Build history of the part. All positions in model axes, mm. A direction names the side the tool comes from. Coordinates: 2 decimals unless noted, no trailing zeros. Write each loop counter-clockwise with the first axis right and the second up, starting at its lowest first coordinate (ties: lowest second). Pieces come first, ordered by that corner, then holes.
```python
from build123d import *
from build123d.topology import SkipClean

# Parameters (mm, degrees)
SKETCH_1_R          = 12.5
EXTRUDE_1_DEPTH     = 4
SKETCH_2_R          = 1
EXTRUDE_2_DEPTH     = 7.5
SKETCH_5_R          = 6
CUT_EXTRUDE_1_DEPTH = 10
CUT_EXTRUDE_START   = -7.5
SKETCH_7_R          = 1
CUT_EXTRUDE_2_DEPTH = 7.5
SKETCH_8_R          = 12.5
SKETCH_8_R_2        = 6
CUT_EXTRUDE_3_DEPTH = 10
SKETCH_9_R          = 1
EXTRUDE_3_DEPTH     = 10
CUT_EXTRUDE_START_2 = -14
SKETCH_10_R         = 1
CUT_EXTRUDE_4_DEPTH = 14
SKETCH_11_R         = 8
CUT_EXTRUDE_5_DEPTH = 10
EXTRUDE_START       = -10
SKETCH_12_R         = 8
EXTRUDE_4_DEPTH     = 10
SKETCH_14_R         = 8
CUT_EXTRUDE_6_DEPTH = 10
SKETCH_15_W         = 0.086708075
SKETCH_15_H         = 4
SKETCH_16_R         = 0.7
CUT_EXTRUDE_7_DEPTH = 10
SKETCH_18_R         = 12.5
EXTRUDE_5_DEPTH     = 2.07
CUT_EXTRUDE_START_3 = -2.07
SKETCH_20_R         = 8
CUT_EXTRUDE_8_DEPTH = 2.07


with BuildPart() as part:
    # 草图1 → 凸台-拉伸1 (new body)
    with BuildSketch(Plane(origin=(0, 0, 0), x_dir=(1, 0, 0), z_dir=(0, 1, 0))):
        with Locations(Location((0, 0, 0), (0, 0, 270))):
            Circle(SKETCH_1_R)
    extrude(amount=EXTRUDE_1_DEPTH)

    # 草图2 → 凸台-拉伸2 (add)
    with BuildSketch(Plane(origin=(0, 4, 0), x_dir=(1, 0, 0), z_dir=(0, 1, 0))):
        with Locations(Location((10, 0, 0), (0, 0, 270))):
            Circle(SKETCH_2_R)
        with Locations(Location((3.399186938, -10.461621679, 0), (0, 0, 270))):
            Circle(SKETCH_2_R)
        with Locations(Location((-8.590169944, -7.416694292, 0), (0, 0, 270))):
            Circle(SKETCH_2_R)
        with Locations(Location((-9.399186938, 4.926796007, 0), (0, 0, 270))):
            Circle(SKETCH_2_R)
        with Locations(Location((2.090169944, 9.510565163, 0), (0, 0, 270))):
            Circle(SKETCH_2_R)
    extrude(amount=EXTRUDE_2_DEPTH)

    # 草图5 → 切除-拉伸1 (cut)
    with BuildSketch(Plane(origin=(0, 4, 0), x_dir=(1, 0, 0), z_dir=(0, 1, 0))):
        with Locations(Location((0, 0, 0), (0, 0, 270))):
            Circle(SKETCH_5_R)
    extrude(amount=-CUT_EXTRUDE_1_DEPTH, mode=Mode.SUBTRACT)

    # 草图7 → 切除-拉伸2 (cut)
    with BuildSketch(Plane(origin=(0, 11.5, 0), x_dir=(1, 0, 0), z_dir=(0, 1, 0)).offset(CUT_EXTRUDE_START)):
        with Locations((-9.399186938, 4.926796007)):
            Circle(SKETCH_7_R)
    extrude(amount=CUT_EXTRUDE_2_DEPTH, mode=Mode.SUBTRACT)

    # 草图8 → 切除-拉伸3 (cut)
    with BuildSketch(Plane(origin=(0, 4, 0), x_dir=(1, 0, 0), z_dir=(0, 1, 0))):
        with Locations(Location((0, 0, 0), (0, 0, 270))):
            Circle(SKETCH_8_R)
        with Locations(Location((0, 0, 0), (0, 0, 270))):
            Circle(SKETCH_8_R_2, mode=Mode.SUBTRACT)
    extrude(amount=CUT_EXTRUDE_3_DEPTH, mode=Mode.SUBTRACT)

    # 草图9 → 凸台-拉伸3 (add)
    with BuildSketch(Plane(origin=(0, 4, 0), x_dir=(1, 0, 0), z_dir=(0, 1, 0))):
        with Locations(Location((11, 0, 0), (0, 0, 270))):
            Circle(SKETCH_9_R)
        with Locations(Location((3.399186938, -10.461621679, 0), (0, 0, 270))):
            Circle(SKETCH_9_R)
        with Locations(Location((-8.899186938, -6.465637775, 0), (0, 0, 270))):
            Circle(SKETCH_9_R)
        with Locations(Location((-8.899186938, 6.465637775, 0), (0, 0, 270))):
            Circle(SKETCH_9_R)
        with Locations(Location((3.399186938, 10.461621679, 0), (0, 0, 270))):
            Circle(SKETCH_9_R)
    extrude(amount=EXTRUDE_3_DEPTH)

    # 草图10 → 切除-拉伸4 (cut)
    with BuildSketch(Plane(origin=(0, 14, 0), x_dir=(1, 0, 0), z_dir=(0, 1, 0)).offset(CUT_EXTRUDE_START_2)):
        with Locations(Location((-8.899186938, -6.465637775, 0), (0, 0, 270))):
            Circle(SKETCH_10_R)
        with Locations(Location((3.399186938, -10.461621679, 0), (0, 0, 270))):
            Circle(SKETCH_10_R)
        with Locations(Location((11, 0, 0), (0, 0, 270))):
            Circle(SKETCH_10_R)
        with Locations(Location((3.399186938, 10.461621679, 0), (0, 0, 270))):
            Circle(SKETCH_10_R)
        with Locations(Location((-8.899186938, 6.465637775, 0), (0, 0, 270))):
            Circle(SKETCH_10_R)
    extrude(amount=CUT_EXTRUDE_4_DEPTH, mode=Mode.SUBTRACT)

    # 草图11 → 切除-拉伸5 (cut)
    with BuildSketch(Plane(origin=(0, 4, 0), x_dir=(1, 0, 0), z_dir=(0, 1, 0))):
        with Locations(Location((0, 0, 0), (0, 0, 270))):
            Circle(SKETCH_11_R)
    extrude(amount=-CUT_EXTRUDE_5_DEPTH, mode=Mode.SUBTRACT)

    # 草图12 → 凸台-拉伸4 (add)
    # profile 1 of 2: a face of its own
    with BuildSketch(Plane(origin=(0, 4, 0), x_dir=(1, 0, 0), z_dir=(0, 1, 0)).offset(EXTRUDE_START)):
        with BuildLine():
            ThreePointArc((8.48540775, 9.178663046), (2.781152949, 8.559508647), (-1.469756299, 12.413291925))
            ThreePointArc((-1.469756299, 12.413291925), (-3.86271243, 11.888206454), (-6.107292102, 10.906465201))
            ThreePointArc((-6.107292102, 10.906465201), (-7.281152949, 5.290067271), (-12.259921848, 2.438096855))
            ThreePointArc((-12.259921848, 2.438096855), (-12.5, 0), (-12.259921848, -2.438096855))
            ThreePointArc((-12.259921848, -2.438096855), (-7.281152949, -5.290067271), (-6.107292102, -10.906465201))
            ThreePointArc((-6.107292102, -10.906465201), (-3.86271243, -11.888206454), (-1.469756299, -12.413291925))
            ThreePointArc((-1.469756299, -12.413291925), (2.781152949, -8.559508647), (8.48540775, -9.178663046))
            ThreePointArc((8.48540775, -9.178663046), (10.11271243, -7.347315654), (11.3515625, -5.233739467))
            ThreePointArc((11.3515625, -5.233739467), (9, 0), (11.3515625, 5.233739467))
            ThreePointArc((11.3515625, 5.233739467), (10.11271243, 7.347315654), (8.48540775, 9.178663046))
        make_face()
        Circle(SKETCH_12_R, mode=Mode.SUBTRACT)
    # profile 2 of 2: a face of its own
    with BuildSketch(Plane(origin=(0, 4, 0), x_dir=(1, 0, 0), z_dir=(0, 1, 0)).offset(EXTRUDE_START)):
        Circle(SKETCH_12_R)
    extrude(amount=EXTRUDE_4_DEPTH)

    # 草图14 → 切除-拉伸6 (cut)
    with SkipClean():  # the faces are left unmerged after this step: merging them gives an invalid solid
        with BuildSketch(Plane.XZ.offset(6)):
            with Locations(Location((0, 0, 0), (0, 0, 270))):
                Circle(SKETCH_14_R)
        extrude(amount=-CUT_EXTRUDE_6_DEPTH, mode=Mode.SUBTRACT)
    add(part.part.scale(1), mode=Mode.REPLACE)  # the faces are merged on a copy

    # 草图15 → 切除-旋转2 (revolve, cut)
    with BuildSketch(Plane(origin=(0, 0, 0), x_dir=(0, 0, -1), z_dir=(1, 0, 0)), mode=Mode.PRIVATE) as cut_revolve_2_sk:
        with Locations((12.456645963, -3)):
            Rectangle(SKETCH_15_W, SKETCH_15_H)
        Polygon((12.413291925, -1), (12.413291925, -5), (9.178663046, -3.93256933), (9.178663046, -2.06743067), align=None)
    revolve(cut_revolve_2_sk.sketch.rotate(Axis((0, 0, 0), (0, -1, 0)), 353.247512934), axis=Axis((0, 0, 0), (0, -1, 0)), mode=Mode.SUBTRACT)

    # 草图16 → 切除-拉伸7 (cut)
    with BuildSketch(Plane(origin=(0, 0, 0), x_dir=(0, 0, -1), z_dir=(1, 0, 0))):
        with Locations((0, -3)):
            Circle(SKETCH_16_R)
    extrude(amount=-CUT_EXTRUDE_7_DEPTH, mode=Mode.SUBTRACT)

    # 草图17 → 切除-旋转4 (revolve, cut)
    with BuildSketch(Plane(origin=(0, 0, 0), x_dir=(0, 0, -1), z_dir=(1, 0, 0)), mode=Mode.PRIVATE) as cut_revolve_4_sk:
        Polygon((12.5, -1), (9.265914401, -2.06743067), (8.289016568, -2.06743067), (12.5, 0), align=None)
    revolve(cut_revolve_4_sk.sketch.rotate(Axis((0, 0, 0), (0, 1, 0)), 6.752487066), axis=Axis((0, 0, 0), (0, 1, 0)), mode=Mode.SUBTRACT)

    # 草图18 → 凸台-拉伸5 (add)
    with SkipClean():  # the faces are left unmerged after this step: merging them gives an invalid solid
        with BuildSketch(Plane.XZ.offset(6)):
            with Locations(Location((0, 0, 0), (0, 0, 263.247512934))):
                Circle(SKETCH_18_R)
        extrude(amount=-EXTRUDE_5_DEPTH)

    # 草图19 → 切除-旋转5 (revolve, cut)
    with SkipClean():  # the faces are left unmerged after this step: merging them gives an invalid solid
        with BuildSketch(Plane(origin=(0, 0, 0), x_dir=(0, 0, -1), z_dir=(1, 0, 0))):
            Polygon((12.5, -2.06743067), (12.5, -4.965), (8.289016568, -3.93), (8.289016568, -2.06743067), align=None)
        revolve(axis=Axis((0, 0, 0), (0, 1, 0)), mode=Mode.SUBTRACT)

    # 草图20 → 切除-拉伸8 (cut)
    with SkipClean():  # the faces are left unmerged after this step: merging them gives an invalid solid
        with BuildSketch(Plane(origin=(0, -3.93, 0), x_dir=(1, 0, 0), z_dir=(0, 1, 0)).offset(CUT_EXTRUDE_START_3)):
            with Locations(Location((0, 0, 0), (0, 0, 90))):
                Circle(SKETCH_20_R)
        extrude(amount=CUT_EXTRUDE_8_DEPTH, mode=Mode.SUBTRACT)


solid = part.part
```
1. Saw through at C-C on y = 2.5. List the corners of the cut face in (x, z).
Computed values:
outline: circle Ø25 at (0, 0); hole circle Ø2 at (-8.9, -6.47); hole circle Ø2 at (-8.9, 6.47); hole circle Ø16 at (0, 0); hole circle Ø2 at (3.4, -10.46); hole circle Ø2 at (3.4, 10.46); hole circle Ø2 at (11, 0)
2. Saw through at D-D on z = -10.5. State how many separate pieces and enclosed holes the cut face has, plus the area to 3 significant figures.
Computed values:
separate pieces: 3
enclosed holes: 0
area: 68.7 mm2
3. Saw through at A-A on z = 0. List the corners of the cut face in (x, y) (3 decimals), plus the area to 3 significant figures.
Computed values:
outline: (-12.5, -6) - (-8, -6) - (-8, -3.7) - (-8.289, -3.7) - (-8.289, -3.93) - (-12.5, -4.965) - close; (-12.5, 0) - (-8.289, -2.067) - (-8.289, -2.3) - (-8, -2.3) - (-8, 4) - (-12.5, 4) - close; (8, -6) - (12.5, -6) - (12.5, -4.965) - (8.289, -3.93) - (8.289, -2.067) - (9, -1.718) - (9, 0) - (10, 0) - (10, 4) - (8, 4) - close; (12, 0) - (12.5, 0) - (12.5, 4) - (12, 4) - close
area: 49.8 mm2
4. Mould opens along Y. For faces 1 (the face through (-8.1, -6, 1.1)), 2 (the face through (3.44, 1.97, -11.46)), 3 (the face through (2.86, -0.68, -8.534)) say: +Y half, -Y half, draft (parallel to the pull), parting line (faces both ways), or undercut.
Computed values:
face 1: -Y half
face 2: draft
face 3: undercut
5. 3-axis set-ups, long thin cutter, end or side, ignore diameter. For faces 4 (the face through (4, 0, 9)), 5 (the face through (4, 0, -9)), 6 (the face through (9, -1, 0)), 7 (the face through (-8.855, 1.972, 5.467)), 8 (the face through (8.29, -3.98, 1.84)): which of +Z, -Z, +X, -X, +Y, -Y reach the whole face in a straight line?
Computed values:
face 4: +Z
face 5: -Z
face 6: +X
face 7: +Y
face 8: none
6. Flat gauge pins, fed straight in: pin 1 (1.1 mm diameter, centred on y = -3, z = 0, fed in from +X); pin 2 (2 mm diameter, centred on x = 5.5, y = 2.5, fed in from +Z); pin 3 (4 mm diameter, centred on y = 1, z = -4.5, fed in from +X). Where does each tip first touch, or does it go through?
Computed values:
pin 1: stops at x = 8.29
pin 2: stops at z = 11.66
pin 3: stops at x = 12.25
7. Probe line 1 along X through (y, z) = (2, 6.75); line 2 along X through (y, z) = (0.5, -7); line 3 along Z through (x, y) = (3.5, 0.5). List the from-to ranges inside material, lowest first.
Computed values:
line 1: x = -10.52 to -9.86, -7.94 to -4.29, 4.29 to 10.52
line 2: x = -10.36 to -9.74, -8.05 to -3.87, 3.87 to 10.36
line 3: z = -12 to -11.46, -9.47 to -7.19, 7.19 to 9.47, 11.46 to 12
8. Saw through at B-B on x = 0. List the corners of the cut face in (y, z) (3 decimals).
Computed values:
outline: (-6, -12.5) - (-4.965, -12.5) - (-3.93, -8.289) - (-2.067, -8.289) - (-1.099, -10.262) - (0, -10.262) - (0, -12.5) - (4, -12.5) - (4, -8) - (-6, -8) - close; (-6, 8) - (4, 8) - (4, 12.5) - (0, 12.5) - (0, 10.262) - (-1.099, 10.262) - (-2.067, 8.289) - (-3.93, 8.289) - (-4.965, 12.5) - (-6, 12.5) - close
